Part model, mm, in its own coordinate system. Face numbers are marked on the shaded views. A direction names the side the tool comes from. Give positions to 0.01 mm unless a question says otherwise; leave off trailing zeros. Order: outer loops, then holes, each group sorted by start corner. A loop starts at its lowest first (then second) coordinate and runs counter-clockwise, first axis right, second up. Notation, with made-up numbers: (33.5, 75.25) - (75.5, 75.25) arc R28 cw to (75.5, 99.25) - close; hole circle Ø11 at (-31, 0.25). An arc over 180 degrees is marked (long way). One line per item, written item: value.
Autodesk Inventor part; units mm, degrees
ref_plane "YZ Plane" through (0, 0, 0) normal (1, 0, 0) x (0, 1, 0)
ref_plane "XZ Plane" through (0, 0, 0) normal (0, 1, 0) x (-1, 0, 0)
ref_plane "XY Plane" through (0, 0, 0) normal (0, 0, 1) x (1, 0, 0)
sketch "Skizze1" plane through (0, 0, 0) normal (0, 0, 1) x (1, 0, 0)
  circle A0 centre (0, 0) radius 1
  dimension "d0" = 2
extrude "Extrusion1" add sketch "Skizze1" along normal blind 0.5
sketch "Skizze2" plane through (0, 0, 0.5) normal (0, 0, 1) x (1, 0, 0)
  circle A0 centre (0, 0) radius 0.75
  dimension "d3" = 1.5
extrude "Extrusion2" add sketch "Skizze2" along normal blind 8.5
sketch "Skizze3" plane through (0, 0, 9) normal (0, 0, 1) x (1, 0, 0)
  circle A0 centre (0, 0) radius 0.45
  dimension "d6" = 0.9
extrude "Extrusion3" add sketch "Skizze3" along normal blind 3
fillet "Rundung1" radius 0.45 1 edges at (-0.45, 0, 12)
sketch "Skizze4" plane through (0, 0, 0) normal (0, 0, -1) x (-1, 0, 0)
  circle A0 centre (0, 0) radius 0.45
  dimension "d10" = 0.9
extrude "Extrusion4" add sketch "Skizze4" along normal blind 2
properties part number "PoGo_pin" material "Gold"
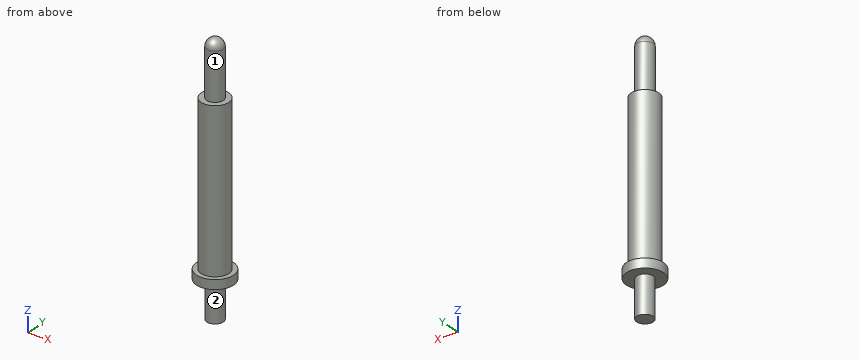
1) Which spindle directions (+Z, -Z, +X, -X, +Y, -Y) get a long thin tool onto all of the face, cutting with end or side? Do the marked faces 1 and 2. Say none if no direction does.
Answer:
face 1: +Z
face 2: -Z
2) Slice it at D-D on y = -0.6. Write the cut outline in (x, z), then the cut area to 3 significant figures.
Answer:
outline: (-0.8, 0) - (0.8, 0) - (0.8, 0.5) - (0.45, 0.5) - (0.45, 9) - (-0.45, 9) - (-0.45, 0.5) - (-0.8, 0.5) - close
area: 8.45 mm2
3) Slice it at A-A on y = 0. Write the cut outline in (x, z), then the cut area to 3 significant figures.
Answer:
outline: (-1, 0) - (-0.45, 0) - (-0.45, -2) - (0.45, -2) - (0.45, 0) - (1, 0) - (1, 0.5) - (0.75, 0.5) - (0.75, 9) - (0.45, 9) - (0.45, 11.55) arc R0.45 ccw to (-0.45, 11.55) - (-0.45, 9) - (-0.75, 9) - (-0.75, 0.5) - (-1, 0.5) - close
area: 18.2 mm2
4) Wall check: line 1 along Z through (x, y) = (-0.2, -0.45); line 2 along Z through (x, y) = (-0.75, 0.25); line 3 along Y through (x, z) = (0.6, 6). Give the ranges that are in metal, low to high. Write a range as [from, to].
Answer:
line 1: z = [0, 9]
line 2: z = [0, 0.5]
line 3: y = [-0.45, 0.45]
5) Drop a flat-ended pin along its axis: P1, Ø1, axis at x = 0, y = -0.5, coming from the -Z side. Give the stop position or say it passes through.
Answer:
P1: stops at z = -2
6) Slice it at C-C on z = 4.75. Write the cut outline in (x, y), then the cut area to 3 significant figures.
Answer:
outline: circle Ø1.5 at (0, 0)
area: 1.77 mm2
